Geometry check sheet. Reference: the model listing, model coordinates, mm. Face numbers are marked on the shaded views. Give positions to 0.01 mm unless a question says otherwise; leave off trailing zeros. Write each loop counter-clockwise with the first axis right and the second up, starting at its lowest first coordinate (ties: lowest second). Pieces come first, ordered by that corner, then holes. Notation, with made-up numbers: (-20.5, 7) - (-3.5, 7) arc R26 ccw to (-3.5, 37) - close; hole circle Ø6 at (24, -9). An arc over 180 degrees is marked (long way). Write item = value, one per line. Start each with the question number.
(1) Draft check along Z on the marked faces 1, 2 and 3. Enter one of: pulls with the +Z half, pulls with the -Z half, needs draft (parallel to the pull), parting line crosses it, or undercut.
(2) Thickness scan on L1, parallel to Z at x = 5.5, y = 18.25; L2, parallel to Z at x = -1, y = 17.25; L3, parallel to Y at x = 3, z = 6.75. Record the ranges inside material, lowest first.
(3) Depth check by flat-ended pin: pin 1 Ø6 at (x, z) = (6, 6) entering from -Y; pin 2 Ø3 at (x, z) = (-6.5, 2) entering from -Y; pin 3 Ø2 at (x, y) = (6, 19.5) entering from +Z. Enter the tip coordinate at first touch or a pass-through.
(4) Section check A-A, the plane y = 22.5. Enter the section's corners in (x, z).
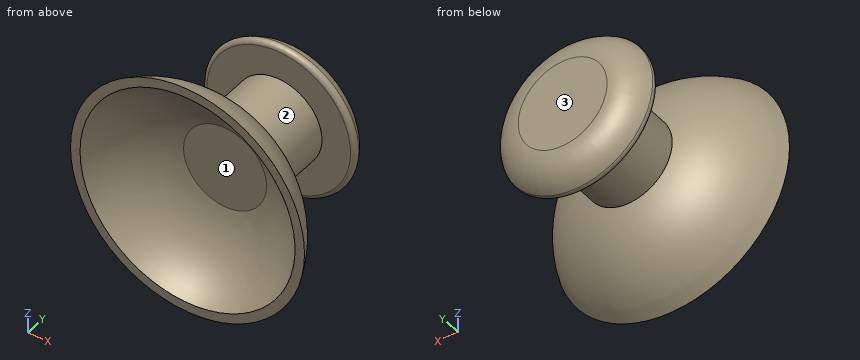
```python
from build123d import *

# Parameters (mm, degrees)
FILLET1_R = 0.5


with BuildPart() as part:
    # Sketch1 → Revolve1 (revolve)
    with BuildSketch(Plane.XY):
        with BuildLine():
            Line((0, 31.617857892), (0, 20.022445397))
            Line((0, 20.022445397), (-4.789317778, 20.022445397))
            ThreePointArc((-4.789317778, 20.022445397), (-9.296235454, 17.896468434), (-12.402618998, 14))
            Line((-12.402618998, 14), (-13.5, 14))
            ThreePointArc((-13.5, 14), (-10.100300372, 18.532507594), (-5, 21))
            Line((-5, 21), (-5, 28.617857892))
            Line((-5, 28.617857892), (-9, 28.617857892))
            ThreePointArc((-9, 28.617857892), (-7.576506397, 30.780135552), (-5.127016654, 31.617857892))
            Line((-5.127016654, 31.617857892), (0, 31.617857892))
        make_face()
    revolve(axis=Axis((0, 31.617857892, 0), (0, -1, 0)))

    # Fillet1
    fillet1_edges = [part.edges().sort_by_distance(p)[0] for p in [
        (9, 28.617857892, 0),
    ]]
    fillet(fillet1_edges, radius=FILLET1_R)


solid = part.part
```
Model answer:
q1.face_1 = undercut
q1.face_2 = parting line crosses it
q1.face_3 = needs draft
q2.L1 = -8.86 to -6.9, 6.9 to 8.86
q2.L2 = -11.39 to -9.99, 9.99 to 11.39
q2.L3 = 19.11 to 20.22, 28.62 to 30.92
q3.pin_1 = 15.57
q3.pin_2 = 18.6
q3.pin_3 = 8.33
q4.outline = circle Ø10 at (0, 0)
